Build history of the part. All positions in model axes, mm. Face numbers are marked on the shaded views. Coordinates: 2 decimals unless noted, no trailing zeros. Order: outer loops, then holes, each group sorted by start corner. A loop starts at its lowest first (then second) coordinate and runs counter-clockwise, first axis right, second up. Notation, with made-up numbers: (87, 18) - (101, 18) arc R22 cw to (101, 50) - close; hole circle Ø5 at (43, 18.5). An arc over 180 degrees is marked (long way). Return JSON: item names as keys, results as strings.
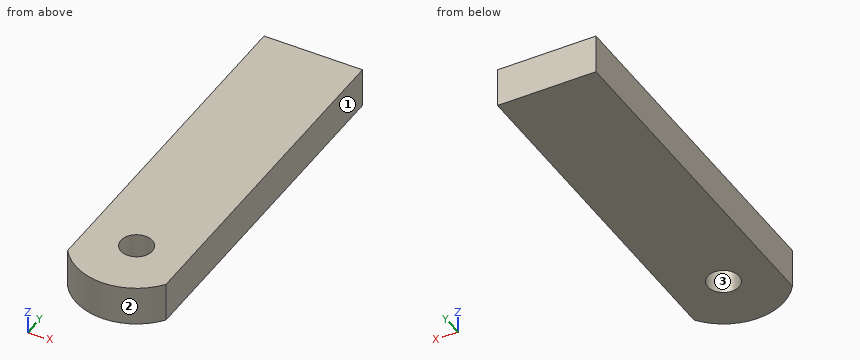
Autodesk Inventor part; units mm, degrees
ref_plane "YZ Plane" through (0, 0, 0) normal (1, 0, 0) x (0, 1, 0)
ref_plane "XZ Plane" through (0, 0, 0) normal (0, 1, 0) x (-1, 0, 0)
ref_plane "XY Plane" through (0, 0, 0) normal (0, 0, 1) x (1, 0, 0)
sketch "Sketch1" plane through (0, 0, 0) normal (0, 0, 1) x (1, 0, 0)
  line L0 (-25, 160) -> (25, 160)
  line L1 (25, 160) -> (25, -18)
  line L2 (-25, 160) -> (-25, -18)
  arc A0 (-25, -18) -> (25, -18) centre (0, 0) ccw
  dimension "d62" = 90
  dimension "d63" = 160
  dimension "d64" = 50
  dimension "d65" = 18
extrude "Extrusion1" add sketch "Sketch1" along normal blind 20
sketch "Sketch10" plane through (0, 0, 0) normal (0, 0, -1) x (-1, 0, 0)
  circle A0 centre (0, 0) radius 8
  dimension "d54" = 16
extrude "Extrusion7" cut sketch "Sketch10" against normal through all
properties part number "Throttle Arm" material "Aluminum 6061-AHC"
1. Probe L1, parallel to X at y = -0.5, z = 9.25; L2, parallel to Y at x = 4.5, z = 15; L3, parallel to Y at x = -9.5, z = 7.5. List the from-to ranges inside material, lowest first.
Check values:
{"L1": "-25 to -7.98, 7.98 to 25", "L2": "-30.48 to -6.61, 6.61 to 160", "L3": "-29.3 to 160"}
2. Cut at B-B on y = 0. Give the cut face in (x, z), plus the area to 3 significant figures.
Check values:
{"outline": "(-25, 0) - (-8, 0) - (-8, 20) - (-25, 20) - close; (8, 0) - (25, 0) - (25, 20) - (8, 20) - close", "area": "680 mm²"}
3. Cut at D-D on x = 16.5. Give the cut face in (y, z), plus the area to 3 significant figures.
Check values:
{"outline": "(-26.01, 0) - (160, 0) - (160, 20) - (-26.01, 20) - close", "area": "3,720 mm²"}
4. Mould opens along Y. For the marked faces 1, 2 and 3 say: pulls with the +Y half, pulls with the -Y half, needs draft (parallel to the pull), parting line crosses it, or undercut.
Check values:
{"face 1": "needs draft", "face 2": "pulls with the -Y half", "face 3": "undercut"}
5. Cut at A-A on x = 0. Give the cut face in (y, z), plus the area to 3 significant figures.
Check values:
{"outline": "(-30.81, 0) - (-8, 0) - (-8, 20) - (-30.81, 20) - close; (8, 0) - (160, 0) - (160, 20) - (8, 20) - close", "area": "3,500 mm²"}
6. Drop a flat-ended pin along its axis: pin 1 (1.5 mm diameter, centred on x = -3.5, y = 67, fed in from -Z). Give the stop position or say it passes through.
Check values:
{"pin 1": "z = 0"}
7. Cut at C-C on z = 17. Give the cut face in (x, y).
Check values:
{"outline": "(-25, -18) arc R30.81 ccw to (25, -18) - (25, 160) - (-25, 160) - close; hole circle Ø16 at (0, 0)"}
